```python
from build123d import *

# Parameters (mm, degrees)
EXTRUDE1_START              = -16
SKETCH1_R                   = 9.128125
EXTRUDE1_DEPTH              = 32
F_3_8_16_TAPPED_HOLE3_D     = 7.9375
F_3_8_16_TAPPED_HOLE3_DEPTH = 14.762
F_3_8_16_TAPPED_HOLE3_TIP   = 2.384665582
F_3_8_16_TAPPED_HOLE4_D     = 7.9375
F_3_8_16_TAPPED_HOLE4_DEPTH = 14.762
F_3_8_16_TAPPED_HOLE4_TIP   = 2.384665582


with BuildPart() as part:
    # Sketch1 → Extrude1 (new body)
    with BuildSketch(Plane.XY.offset(EXTRUDE1_START)):
        Circle(SKETCH1_R)
    extrude(amount=EXTRUDE1_DEPTH)

    # Sketch2 → Cut-Revolve1 (revolve, cut)
    with BuildSketch(Plane(origin=(0, 0, 0), x_dir=(0, 0, -1), z_dir=(1, 0, 0))):
        with BuildLine():
            Line((-6, 13.2625), (-6, 15.153312549))
            Line((-6, 15.153312549), (6, 15.153312549))
            Line((6, 15.153312549), (6, 13.2625))
            ThreePointArc((6, 13.2625), (0, 7.2625), (-6, 13.2625))
        make_face()
    revolve(axis=Axis((0, 0, 16), (0, 0, -1)), mode=Mode.SUBTRACT)

    # 3_8-16 Tapped Hole3
    with Locations(Plane.XY.offset(16)):
        with Locations((0, 0)):
            Hole(F_3_8_16_TAPPED_HOLE3_D / 2, depth=F_3_8_16_TAPPED_HOLE3_DEPTH)
            with Locations((0, 0, -(F_3_8_16_TAPPED_HOLE3_DEPTH + F_3_8_16_TAPPED_HOLE3_TIP / 2))):  # 118° drill point
                Cone(0, F_3_8_16_TAPPED_HOLE3_D / 2, F_3_8_16_TAPPED_HOLE3_TIP, mode=Mode.SUBTRACT)

    # 3_8-16 Tapped Hole4
    with Locations(Plane(origin=(0, 0, -16), x_dir=(-1, 0, 0), z_dir=(0, 0, -1))):
        with Locations((0, 0)):
            Hole(F_3_8_16_TAPPED_HOLE4_D / 2, depth=F_3_8_16_TAPPED_HOLE4_DEPTH)
            with Locations((0, 0, -(F_3_8_16_TAPPED_HOLE4_DEPTH + F_3_8_16_TAPPED_HOLE4_TIP / 2))):  # 118° drill point
                Cone(0, F_3_8_16_TAPPED_HOLE4_D / 2, F_3_8_16_TAPPED_HOLE4_TIP, mode=Mode.SUBTRACT)


solid = part.part
```
For this review, take the finished solid that the model builds, in its own axes (mm). A direction names the side the tool comes from. Round coordinates to 2 decimals unless told otherwise and drop trailing zeros. Order: outer loops, then holes, each group sorted by start corner. A loop starts at its lowest first (then second) coordinate and runs counter-clockwise, first axis right, second up.
Q1. We need section D-D, the plane z = 10. Give the boundary of the cut face in (x, y), plus the area to 3 significant figures.
Findings below:
outline: circle Ø18.26 at (0, 0); hole circle Ø7.94 at (0, 0)
area: 212 mm2
Q2. Insertion check: P1, Ø6.5, axis at x = 0, y = 0, coming from the -Z side; P2, Ø2, axis at x = -1, z = 1.5, coming from the -Y side; P3, Ø5, axis at x = -2.5, y = 2.5, coming from the -Z side; P4, Ø5, axis at y = 3, z = -10.5, coming from the +X side. Each pin has a flat end and moves straight along its axis. Give the tip position at first contact, or say it passes through.
Findings below:
P1: stops at z = -0.81
P2: stops at y = -7.76
P3: stops at z = -16
P4: stops at x = 9.11
Q3. We need section A-A, the plane x = 0. Give the boundary of the cut face in (y, z).
Findings below:
outline: (-9.13, -16) - (-3.97, -16) - (-3.97, -1.24) - (-1.91, 0) - (-3.97, 1.24) - (-3.97, 16) - (-9.13, 16) - (-9.13, 4.35) arc R6 cw to (-9.13, -4.35) - close; (1.91, 0) - (3.97, -1.24) - (3.97, -16) - (9.13, -16) - (9.13, -4.35) arc R6 cw to (9.13, 4.35) - (9.13, 16) - (3.97, 16) - (3.97, 1.24) - close
Q4. Wall thickness on line 1 (Y direction, x = 0, z = 9.25); line 2 (Z direction, x = 6, y = 5.25): over which ranges is each line inside the solid? List them lowest first.
Findings below:
line 1: y = -9.13 to -3.97, 3.97 to 9.13
line 2: z = -16 to -2.83, 2.83 to 16
Q5. Machinability: for faces 4 (the cylindrical face through (8.707, 2.742, -10.256)), 5 (the cylindrical face through (0.86, -3.874, 8.516)), which of the approach directions +Z, -Z, +X, -X, +Y, -Y give a long, thin tool a straight path to every point of the face, cutting with its end or side? Answer none if there is none.
Findings below:
face 4: +Z, -Z
face 5: +Z
Q6. We need section C-C, the plane z = 2.5. Give the boundary of the cut face in (x, y), plus the area to 3 significant figures.
Findings below:
outline: circle Ø15.62 at (0, 0); hole circle Ø7.94 at (0, 0)
area: 142 mm2
Q7. Mouldability with a two-part tool opening along X and no side actions: class faces 1 (the cylindrical face through (8.707, 2.742, 10.093)), 2 (the flat face through (2, -4, -16)), 3 (the cylindrical face through (-0.86, -3.874, -8.516)) as pulls with the +X half, pulls with the -X half, needs draft (parallel to the pull), parting line crosses it, or undercut.
Findings below:
face 1: parting line crosses it
face 2: needs draft
face 3: undercut
